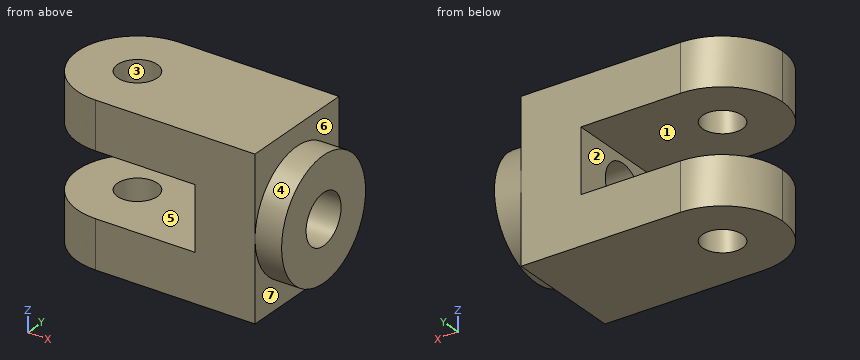
```python
from build123d import *

# Parameters (mm, degrees)
SKETCH1_W           = 132
SKETCH1_H           = 72
BOSS_EXTRUDE1_DEPTH = 95.55
CUT_EXTRUDE3_START  = -95.55
CUT_EXTRUDE3_DEPTH  = 95.55
SKETCH3_W           = 96
SKETCH3_H           = 38.1
CUT_EXTRUDE4_DEPTH  = 137.637485706
SKETCH4_R           = 15
CUT_EXTRUDE5_DEPTH  = 167.88260095
BOSS_EXTRUDE2_START = 16
SKETCH5_R           = 36
SKETCH5_R_2         = 15
BOSS_EXTRUDE2_DEPTH = 16
SKETCH6_R           = 12
CUT_EXTRUDE6_DEPTH  = 131.957254476


# Read off the part's stored shape, not the designer's step: Cut-Extrude3
with BuildPart() as part:
    # Sketch1 → Boss-Extrude1 (new body)
    with BuildSketch(Plane.XY):
        Rectangle(SKETCH1_W, SKETCH1_H)
    extrude(amount=BOSS_EXTRUDE1_DEPTH)

    # Cut-Extrude3 outline → Cut-Extrude3 (cut)
    with BuildSketch(Plane.XY.offset(95.55).offset(CUT_EXTRUDE3_START)):
        with BuildLine():
            Line((-66, -36), (-30, -36))
            ThreePointArc((-30, -36), (-55.455844123, -25.455844123), (-66, 0))
            Line((-66, 0), (-66, -36))
        make_face()
        with BuildLine():
            Line((-66, 36), (-66, 0))
            ThreePointArc((-66, 0), (-55.455844123, 25.455844123), (-30, 36))
            Line((-30, 36), (-66, 36))
        make_face()
    extrude(amount=CUT_EXTRUDE3_DEPTH, mode=Mode.SUBTRACT)

    # Sketch3 → Cut-Extrude4 (cut, through all)
    with BuildSketch(Plane(origin=(0, 36, 0), x_dir=(1, 0, 0), z_dir=(0, 1, 0))):
        with Locations((-18, -47.92)):
            Rectangle(SKETCH3_W, SKETCH3_H)
    extrude(amount=-CUT_EXTRUDE4_DEPTH, mode=Mode.SUBTRACT)

    # Sketch4 → Cut-Extrude5 (cut, through all)
    with BuildSketch(Plane(origin=(66, 0, 0), x_dir=(0, 0, -1), z_dir=(1, 0, 0))):
        with Locations((-47.775, 0)):
            Circle(SKETCH4_R)
    extrude(amount=-CUT_EXTRUDE5_DEPTH, mode=Mode.SUBTRACT)

    # Sketch5 → Boss-Extrude2 (add)
    with BuildSketch(Plane(origin=(66, 0, 0), x_dir=(0, 0, -1), z_dir=(1, 0, 0)).offset(BOSS_EXTRUDE2_START)):
        with Locations(Location((-47.775, 0, 0), (0, 0, 270))):
            Circle(SKETCH5_R)
        with Locations((-47.775, 0)):
            Circle(SKETCH5_R_2, mode=Mode.SUBTRACT)
    extrude(amount=-BOSS_EXTRUDE2_DEPTH)

    # Sketch6 → Cut-Extrude6 (cut, through all)
    with BuildSketch(Plane(origin=(0, 0, 0), x_dir=(-1, 0, 0), z_dir=(0, 0, -1))):
        with Locations((30, 0)):
            Circle(SKETCH6_R)
    extrude(amount=-CUT_EXTRUDE6_DEPTH, mode=Mode.SUBTRACT)


solid = part.part
```
CAD build for the part. Positions are in the model's coordinates, mm. Face numbers are marked on the shaded views. A direction names the side the tool comes from. Coordinates: 2 decimals unless noted, no trailing zeros. Order: outer loops, then holes, each group sorted by start corner. A loop starts at its lowest first (then second) coordinate and runs counter-clockwise, first axis right, second up. Notation, with made-up numbers: (57.25, 5) - (81.25, 5) arc R10 ccw to (81.25, 19) - close; hole circle Ø9 at (35.5, 85). An arc over 180 degrees is marked (long way). Answer in a Markdown table with one row per item.
1. Slice it at B-B, the plane y = -10. List the corners of the cut face in (x, z).
Answer:
| item | result |
|---|---|
| outline | (-64.58, 0) - (-36.63, 0) - (-36.63, 28.87) - (-64.58, 28.87) - close; (-64.58, 66.97) - (-36.63, 66.97) - (-36.63, 95.55) - (-64.58, 95.55) - close; (-23.37, 0) - (66, 0) - (66, 13.19) - (82, 13.19) - (82, 36.59) - (30, 36.59) - (30, 28.87) - (-23.37, 28.87) - close; (-23.37, 66.97) - (30, 66.97) - (30, 58.96) - (82, 58.96) - (82, 82.36) - (66, 82.36) - (66, 95.55) - (-23.37, 95.55) - close |
2. Slice it at C-C, the plane z = 52. List the corners of the cut face in (x, y), then the cut area to 3 significant figures.
Answer:
| item | result |
|---|---|
| outline | (30, -36) - (66, -36) - (66, -35.75) - (82, -35.75) - (82, -14.39) - (30, -14.39) - close; (30, 14.39) - (82, 14.39) - (82, 35.75) - (66, 35.75) - (66, 36) - (30, 36) - close |
| area | 2,240 mm² |
3. 3-axis set-ups, long thin cutter, end or side, ignore diameter. For the marked faces 4, 5, 6 and 7: which of +Z, -Z, +X, -X, +Y, -Y reach the whole face in a straight line?
Answer:
| item | result |
|---|---|
| face 4 | +X |
| face 5 | -X, +Y, -Y |
| face 6 | +Z, +X |
| face 7 | -Z, +X |
4. Drill centre lines: L1, parallel to Z at x = -18.5, y = -27; L2, parallel to Y at x = -30, z = 20.5; L3, parallel to X at y = -8, z = 32.5. Where is each one in solid material? Low to high. Write a range as from..to.
Answer:
| item | result |
|---|---|
| L1 | 0..28.87, 66.97..95.55 |
| L2 | -36..-12, 12..36 |
| L3 | 30..82 |
5. Slice it at A-A, the plane x = 49. List the corners of the cut face in (y, z) (3 decimals), then the cut area to 3 significant figures.
Answer:
| item | result |
|---|---|
| outline | (-36, 0) - (36, 0) - (36, 95.55) - (-36, 95.55) - close; hole circle Ø30 at (0, 47.775) |
| area | 6,170 mm² |
6. Pull direction X, two halves, no side cores. Call the marked faces 1, 2 and 3: +X half, -X half, draft (parallel to the pull), parting line (faces both ways), or undercut.
Answer:
| item | result |
|---|---|
| face 1 | draft |
| face 2 | -X half |
| face 3 | undercut |
7. Flat gauge pins, fed straight in: P1, Ø21.5, axis at x = -30, y = 0, coming from the -Z side; P2, Ø1.5, axis at x = -35.5, z = 16, coming from the +Y side; P3, Ø6, axis at y = -19.5, z = 36, coming from the -X side; P4, Ø4, axis at y = -19.5, z = 76, coming from the -X side. Where does each tip first touch, or does it go through?
Answer:
| item | result |
|---|---|
| P1 | through |
| P2 | y = 35.69 |
| P3 | x = 30 |
| P4 | x = -61.46 |
8. Slice it at D-D, the plane x = 12. List the corners of the cut face in (y, z), then the cut area to 3 significant figures.
Answer:
| item | result |
|---|---|
| outline | (-36, 0) - (36, 0) - (36, 28.87) - (-36, 28.87) - close; (-36, 66.97) - (36, 66.97) - (36, 95.55) - (-36, 95.55) - close |
| area | 4,140 mm² |
